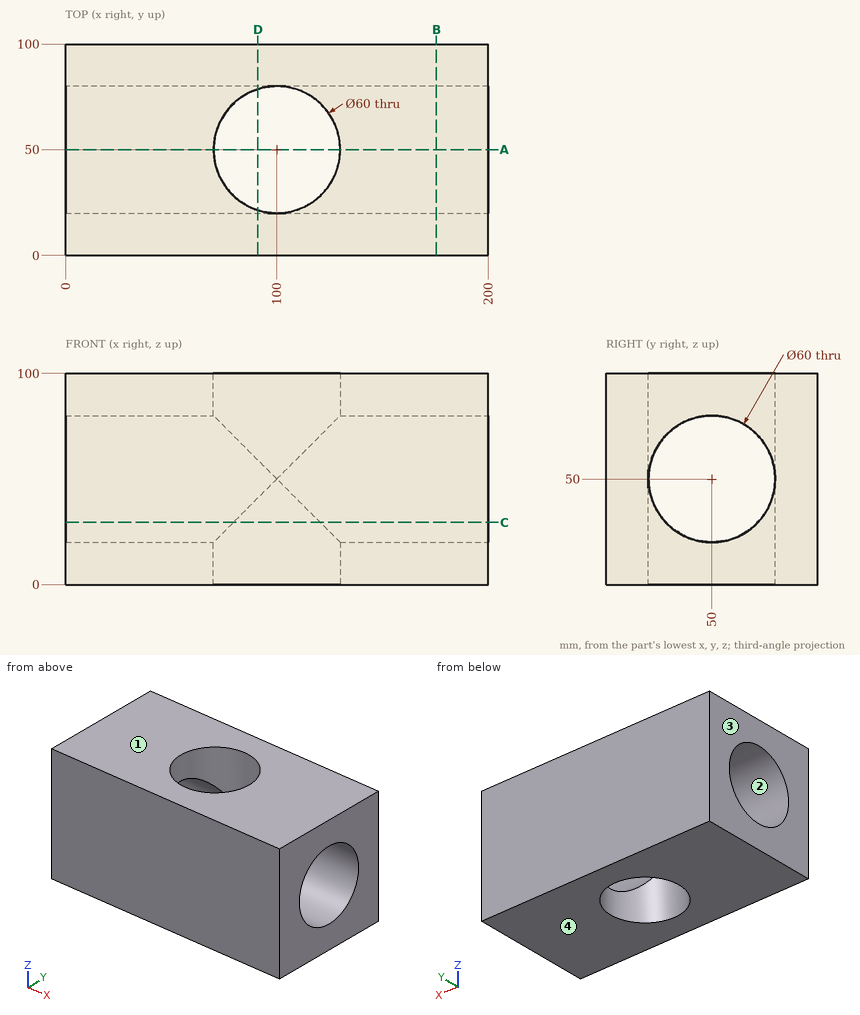
Drawing for the job (mm, zero at the part's lowest x, y, z). Coordinates: 2 decimals unless noted, no trailing zeros. Order: outer loops, then holes, each group sorted by start corner. A loop starts at its lowest first (then second) coordinate and runs counter-clockwise, first axis right, second up. Notation, with made-up numbers: (75.25, -12) -> (126.25, -12) arc R19 cw to (126.25, 24) -> close; hole circle Ø8 at (40.5, 74.25). An arc over 180 degrees is marked (long way). One line per item, written item: value.
(1) Mould opens along Z. For the marked faces 1, 2, 3 and 4 say: pulls with the +Z half, pulls with the -Z half, needs draft (parallel to the pull), parting line crosses it, or undercut.
Checked values:
face 1: pulls with the +Z half
face 2: undercut
face 3: needs draft
face 4: pulls with the -Z half
(2) Slice it at B-B, the plane x = 175.5. List the corners of the cut face in (y, z).
Checked values:
outline: (0, 0) -> (100, 0) -> (100, 100) -> (0, 100) -> close; hole circle Ø60 at (50, 50)
(3) Drop a flat-ended pin along its axis: pin 1 Ø8 at (x, z) = (153, 57.5) entering from -Y. Give the stop position or say it passes through.
Checked values:
pin 1: y = 0
(4) Probe line 1 (Z direction, x = 20, y = 50); line 2 (Z direction, x = 147, y = 38.5). List the from-to ranges inside material, lowest first. Write a range as [from, to].
Checked values:
line 1: [0, 20], [80, 100]
line 2: [0, 22.29], [77.71, 100]
(5) Slice it at A-A, the plane y = 50. List the corners of the cut face in (x, z), plus the area to 3 significant figures.
Checked values:
outline: (0, 0) -> (70, 0) -> (70, 20) -> (0, 20) -> close; (0, 80) -> (70, 80) -> (70, 100) -> (0, 100) -> close; (130, 0) -> (200, 0) -> (200, 20) -> (130, 20) -> close; (130, 80) -> (200, 80) -> (200, 100) -> (130, 100) -> close
area: 5,600 mm2
(6) Slice it at D-D, the plane x = 91. List the corners of the cut face in (y, z).
Checked values:
outline: (0, 0) -> (21.38, 0) -> (21.38, 41) arc R30 cw to (21.38, 59) -> (21.38, 100) -> (0, 100) -> close; (78.62, 0) -> (100, 0) -> (100, 100) -> (78.62, 100) -> (78.62, 59) arc R30 cw to (78.62, 41) -> close
(7) Slice it at C-C, the plane z = 29.5. List the corners of the cut face in (x, y).
Checked values:
outline: (0, 0) -> (200, 0) -> (200, 28.1) -> (120.5, 28.1) arc R30 cw to (79.5, 28.1) -> (0, 28.1) -> close; (0, 71.9) -> (79.5, 71.9) arc R30 cw to (120.5, 71.9) -> (200, 71.9) -> (200, 100) -> (0, 100) -> close
